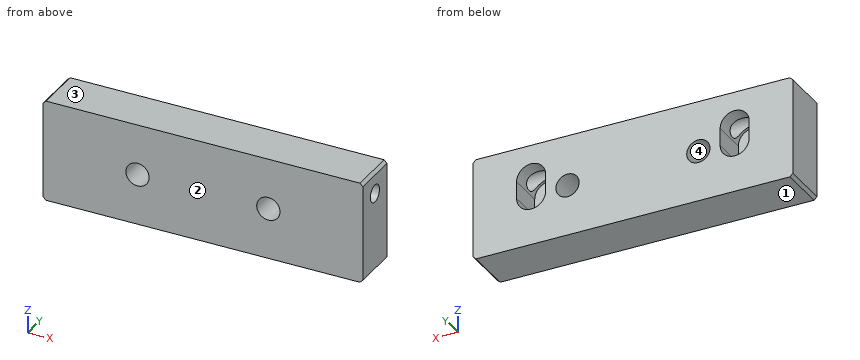
```python
from build123d import *

# Parameters (mm, degrees)
F1_W     = 10
F1_H     = 35.0110880776
F1_W_2   = 90
F1_R     = 5
F2_DEPTH = 16
F3_SIZE  = 1
F7_DEPTH = 12


# Not quite as in the source:
# - a feature of the source that left no trace in its solid (it failed there, or was rolled back) is left out
# - a pattern or mirror of a feature is missing from the dataset's text; its kind, count and spacing are read off the source's solid


with BuildPart() as f2:
    # F1 (on Front) → F2 (new body)
    with BuildSketch(Plane.XZ):
        with Locations((-50, 0)):
            Rectangle(F1_W, F1_H)
        Rectangle(F1_W_2, F1_H)
        with Locations((-35, 0)):
            Circle(F1_R, mode=Mode.SUBTRACT)
        with BuildLine():
            ThreePointArc((-26.5, 0), (-22.5, 4), (-18.5, 0))
            ThreePointArc((-18.5, 0), (-22.5, -4), (-26.5, 0))
        make_face(mode=Mode.SUBTRACT)
        with BuildLine():
            ThreePointArc((26.5, 0), (22.5, -4), (18.5, 0))
            ThreePointArc((18.5, 0), (22.5, 4), (26.5, 0))
        make_face(mode=Mode.SUBTRACT)
        with BuildLine():
            ThreePointArc((40, 0), (35, -5), (30, 0))
            ThreePointArc((30, 0), (35, 5), (40, 0))
        make_face(mode=Mode.SUBTRACT)
        with Locations((-35, 0)):
            Circle(F1_R)
        with BuildLine():
            ThreePointArc((40, 0), (35, 5), (30, 0))
            ThreePointArc((30, 0), (35, -5), (40, 0))
        make_face()
        with Locations((50, 0)):
            Rectangle(F1_W, F1_H)
    extrude(amount=-F2_DEPTH)

    # F3
    f3_edges = [f2.edges().sort_by_distance(p)[0] for p in [
        (55, 8, -17.505544),
        (55, 8, 17.505544),
        (-55, 8, -17.505544),
        (-55, 8, 17.505544),
    ]]
    chamfer(f3_edges, length=F3_SIZE)

    # F4 (on offset) → F5 (revolve, cut)
    with BuildSketch(Plane.XY.offset(10)):
        Polygon((57.6581534887, 5), (57.6581534887, 8), (-50, 8), (-48.1974181429, 5), align=None)
    revolve(axis=Axis((3.8290767443, 8, 10), (-1, 0, 0)), mode=Mode.SUBTRACT)

    # F6 (on face) → F7 (cut)
    with BuildSketch(Plane(origin=(0, 16, 0), x_dir=(-1, 0, 0), z_dir=(0, 1, 0))):
        with BuildLine():
            Line((30, 6), (30, 0))
            ThreePointArc((30, 0), (35, -5), (40, 0))
            Line((40, 0), (40, 6))
            ThreePointArc((40, 6), (35, 11), (30, 6))
        make_face()
    f7 = extrude(amount=-F7_DEPTH, mode=Mode.SUBTRACT)

    # F7_copies: F7 across plane
    add(f7.mirror(Plane(origin=(0, 0, 0), x_dir=(0, 0, 1), z_dir=(1, 0, 0))), mode=Mode.SUBTRACT)


solid = f2.part
```
CAD build for the part. Positions are in the model's coordinates, mm. Face numbers are marked on the shaded views. Round coordinates to 2 decimals unless told otherwise and drop trailing zeros. Order: outer loops, then holes, each group sorted by start corner. A loop starts at its lowest first (then second) coordinate and runs counter-clockwise, first axis right, second up. Notation, with made-up numbers: (74.25, 75) - (96.25, 75) arc R14 cw to (96.25, 98) - close; hole circle Ø10 at (40.25, 42.5). An arc over 180 degrees is marked (long way). Answer in a Markdown table with one row per item. Add a question column.
(1) Band-saw the part on D-D on x = 35. List the corners of the cut face in (y, z).
(2) Band-saw the part on A-A on x = -22.5. List the corners of the cut face in (y, z), and give its area (3 significant figures).
(3) Band-saw the part on B-B on y = 2.5. List the corners of the cut face in (x, z).
(4) Drop a flat-ended pin along its axis: pin 1 Ø3 at (x, z) = (-34, -0.5) entering from +Y. Give the stop position or say it passes through.
(5) Band-saw the part on C-C on z = 2. List the corners of the cut face in (x, y), and give its area (3 significant figures).
(6) Mould opens along Z. For the marked faces 1, 2, 3 and 4 say: +Z half, -Z half, draft (parallel to the pull), parting line (faces both ways), or undercut.
(7) Probe L1, parallel to Z at x = -22.5, y = 4.5; L2, parallel to X at y = 9.5, z = 3.5; L3, parallel to Z at x = -13, y = 8. List the from-to ranges inside material, lowest first. Write a range as [from, to].
Data:
| question | item | result |
|---|---|---|
| 1 | outline | (0, -17.51) - (16, -17.51) - (16, -5) - (4, -5) - (4, 11) - (5.17, 11) arc R3 cw to (10.83, 11) - (16, 11) - (16, 17.51) - (0, 17.51) - close |
| 2 | outline | (0, -17.51) - (16, -17.51) - (16, -4) - (0, -4) - close; (0, 4) - (16, 4) - (16, 17.51) - (0, 17.51) - close; hole circle Ø6 at (8, 10) |
| 2 | area | 404 mm^2 |
| 3 | outline | (-55, -16.51) - (-54, -17.51) - (54, -17.51) - (55, -16.51) - (55, 16.51) - (54, 17.51) - (-54, 17.51) - (-55, 16.51) - close; hole circle Ø8 at (-22.5, 0); hole circle Ø8 at (22.5, 0) |
| 4 | pin 1 | stops at y = 4 |
| 5 | outline | (-55, 0) - (-25.96, 0) - (-25.96, 16) - (-30, 16) - (-30, 4) - (-40, 4) - (-40, 16) - (-55, 16) - close; (-19.04, 0) - (19.04, 0) - (19.04, 16) - (-19.04, 16) - close; (25.96, 0) - (55, 0) - (55, 16) - (40, 16) - (40, 4) - (30, 4) - (30, 16) - (25.96, 16) - close |
| 5 | area | 1,300 mm^2 |
| 6 | face 1 | -Z half |
| 6 | face 2 | draft |
| 6 | face 3 | +Z half |
| 6 | face 4 | undercut |
| 7 | L1 | z = [-17.51, -4], [4, 17.51] |
| 7 | L2 | x = [-55, -40], [-30, -24.44], [-20.56, 20.56], [24.44, 30], [40, 55] |
| 7 | L3 | z = [-17.51, 7], [13, 17.51] |
